from build123d import *

# Parameters (mm, degrees)
SKETCH4_R            = 8.5
SKETCH4_R_2          = 4.365
SKETCH4_R_3          = 3.8
SKETCH4_R_4          = 2.4
BOSS_EXTRUDE1_DEPTH  = 2
BOSS_EXTRUDE2_START  = 2
SKETCH4_3_R          = 8.5
SKETCH4_3_R_2        = 4.365
BOSS_EXTRUDE2_DEPTH  = 4
SKETCH4_4_R          = 2.4
CUT_EXTRUDE2_DEPTH   = 18.486852204
CUT_SWEEP1_PROFILE_R = 0.889
SKETCH14_R           = 2.75
SKETCH14_R_2         = 1.75
BOSS_EXTRUDE3_DEPTH  = 6
FILLET3_R            = 4
CHAMFER1_SIZE        = 1


with BuildPart() as part:
    # Sketch1 → Revolve1 (revolve)
    with BuildSketch(Plane(origin=(0, 0, 0), x_dir=(1, 0, 0), z_dir=(0, 1, 0))):
        Polygon((0, 0), (-12.7, 0), (-12.7, 4.365), (-8.73, 4.365), (-7.94, 5.155), (-7.15, 4.365), (-3.97, 4.365), (-3.97, 5.955), (0, 4.365), align=None)
    revolve(axis=Axis((0, 0, 0), (-1, 0, 0)))

    # Sketch4 → Boss-Extrude1 (add)
    # profile 1 of 3: a face of its own
    with BuildSketch(Plane.ZY.offset(12.7)):
        Circle(SKETCH4_R)
        with Locations(Location((0, 0, 0), (0, 0, 180))):
            Circle(SKETCH4_R_2, mode=Mode.SUBTRACT)
    # profile 2 of 3: a face of its own
    with BuildSketch(Plane.ZY.offset(12.7)):
        with Locations(Location((0, 0, 0), (0, 0, 180))):
            Circle(SKETCH4_R_2)
        Circle(SKETCH4_R_3, mode=Mode.SUBTRACT)
    # profile 3 of 3: a face of its own
    with BuildSketch(Plane.ZY.offset(12.7)):
        Circle(SKETCH4_R_3)
        Circle(SKETCH4_R_4, mode=Mode.SUBTRACT)
    extrude(amount=BOSS_EXTRUDE1_DEPTH)

    # Sketch4<3> → Boss-Extrude2 (add)
    with BuildSketch(Plane.ZY.offset(12.7).offset(BOSS_EXTRUDE2_START)):
        Circle(SKETCH4_3_R)
        with Locations(Location((0, 0, 0), (0, 0, 180))):
            Circle(SKETCH4_3_R_2, mode=Mode.SUBTRACT)
    extrude(amount=BOSS_EXTRUDE2_DEPTH)

    # Sketch4<4> → Cut-Extrude2 (cut, through all)
    with BuildSketch(Plane.ZY.offset(12.7)):
        Circle(SKETCH4_4_R)
    extrude(amount=-CUT_EXTRUDE2_DEPTH, mode=Mode.SUBTRACT)

    # Cut-Sweep1: sweep along a path in Sketch5
    with BuildLine(Plane.ZY.offset(18.7)) as cut_sweep1_path:
        CenterArc((0, 0), 6.082351302, 0, 360)
    # Cut-Sweep1 profile (on start of the path) → Cut-Sweep1 (sweep, cut)
    with BuildSketch(Plane(origin=(-18.7, 0, 6.082351302), x_dir=(0, 0, 1), z_dir=(0, 1, 0))):
        Circle(CUT_SWEEP1_PROFILE_R)
    sweep(path=cut_sweep1_path.line, mode=Mode.SUBTRACT)

    # Sketch14 → Boss-Extrude3 (add)
    # profile 1 of 3: a face of its own
    with BuildSketch(Plane.ZY.offset(18.7)):
        with Locations((10.5, 0)):
            Circle(SKETCH14_R)
        with Locations((10.5, 0)):
            Circle(SKETCH14_R_2, mode=Mode.SUBTRACT)
    # profile 2 of 3: a face of its own
    with BuildSketch(Plane.ZY.offset(18.7)):
        with Locations((-5.25, -9.09326674)):
            Circle(SKETCH14_R)
        with Locations((-5.25, -9.09326674)):
            Circle(SKETCH14_R_2, mode=Mode.SUBTRACT)
    # profile 3 of 3: a face of its own
    with BuildSketch(Plane.ZY.offset(18.7)):
        with Locations((-5.25, 9.09326674)):
            Circle(SKETCH14_R)
        with Locations((-5.25, 9.09326674)):
            Circle(SKETCH14_R_2, mode=Mode.SUBTRACT)
    extrude(amount=-BOSS_EXTRUDE3_DEPTH)

    # Fillet3
    # the kernel refuses this fillet: 4 mm, written as the material it adds along each edge
    with BuildSketch(Plane(origin=(-18.7, 8.059160345, -2.701839101), x_dir=(0, 0.13787930988752692, 0.9904490375102291), z_dir=(1, 0, 0))) as fillet3_piece_1:
        with BuildLine():
            CenterArc((3.866081399, -3.931630738), FILLET3_R, 100.608613334, 57.139697136)
            ThreePointArc((0.163964046, -2.4169271), (0.362452033, -1.189436498), (0, 0))
            ThreePointArc((0, 0), (1.564842471, -0.145284682), (3.129684942, 0))
        make_face()
    extrude(amount=6)
    with BuildSketch(Plane(origin=(-18.7, 6.369441471, -5.628518041), x_dir=(0, 0.559831667079214, -0.8286063628378122), z_dir=(1, 0, 0)), Plane(origin=(-18.7, -8.059160345, -2.701839101), x_dir=(0, -0.9975099934945784, -0.07052526411468515), z_dir=(1, 0, 0))) as fillet3_piece_2:
        with BuildLine():
            CenterArc((4.184287724, -3.591105941), FILLET3_R, 116.132681907, 57.139697136)
            ThreePointArc((0.211830564, -3.12250791), (0.250866796, -1.551420461), (0, 0))
            ThreePointArc((0, 0), (1.211241183, -0.281114665), (2.422482367, 0))
        make_face()
    extrude(amount=6)
    with BuildSketch(Plane(origin=(-18.7, -6.369441471, -5.628518041), x_dir=(0, -0.5598316670792142, -0.8286063628378122), z_dir=(1, 0, 0)), Plane(origin=(-18.7, -1.689718874, 8.330357143), x_dir=(0, -0.43767832641536075, 0.8991316269524996), z_dir=(1, 0, 0))) as fillet3_piece_3:
        with BuildLine():
            CenterArc((4.184287724, 3.591105941), FILLET3_R, 186.727620957, 57.139697136)
            ThreePointArc((0.211830564, 3.12250791), (0.250866796, 1.551420461), (0, 0))
            ThreePointArc((0, 0), (1.211241183, 0.281114665), (2.422482367, 0))
        make_face()
    extrude(amount=6)
    with BuildSketch(Plane(origin=(-18.7, 1.689718874, 8.330357143), x_dir=(0, 0.9266936825814681, -0.3758175337362501), z_dir=(1, 0, 0))) as fillet3_piece_4:
        with BuildLine():
            CenterArc((3.866081399, 3.931630738), FILLET3_R, 202.25168953, 57.139697136)
            ThreePointArc((0.163964046, 2.4169271), (0.362452033, 1.189436498), (0, 0))
            ThreePointArc((0, 0), (1.564842471, 0.145284682), (3.129684942, 0))
        make_face()
    extrude(amount=6)

    # Chamfer1
    chamfer1_edges = [part.edges().sort_by_distance(p)[0] for p in [
        (-14.7, 0, -2.4),
    ]]
    chamfer(chamfer1_edges, length=CHAMFER1_SIZE)


solid = part.part
Input: part model. Units: mm. Frame: model coordinates. A direction names the side the tool comes from. Round coordinates to 2 decimals unless told otherwise and drop trailing zeros. Order: outer loops, then holes, each group sorted by start corner. A loop starts at its lowest first (then second) coordinate and runs counter-clockwise, first axis right, second up. Notation, with made-up numbers: (-28, 68.25) - (0, 68.25) arc R10 ccw to (0, 86.25) - close; hole circle Ø8 at (-31.5, 74). An arc over 180 degrees is marked (long way). Answer as a JSON object with one key per item and string values. Group by question number.
(1) Cut plane C-C (y = 0). Count the separate pieces of the cut face and the enclosed holes in it, then the cut area to 3 significant figures.
(2) Material intervals for probe 1 along Y at (x, z) = (-16, -5.25); probe 2 along X at (y, z) = (-4.75, 0) (3 decimals); probe 3 along Z at (x, y) = (-14.75, 1), sorted ascending. Write a range as from..to.
(3) Reachability of faces 5 (the face through (-16.672, -4.328, 0.568)), 6 (the face through (-15.66, -7.39, 4.2)) from +Z, -Z, +X, -X, +Y, -Y: full face, straight path, thin tool, end or side. Return the list, or none.
(4) Draft query along X for faces 1 (the face through (-5.538, -2.95, 3.217)), 2 (the face through (-15.66, 7.33, 4.3)), 3 (the face through (-3.97, -4, 3)), 4 (the face through (0, 2, -2)). Return one class per face: released by +X, released by -X, zero draft, split by the parting line, or undercut.
(5) Pin query (flat end, axial travel): P1, Ø1.5, axis at x = -16, z = 3.5, coming from the +Y side; P2, Ø6, axis at x = -14, z = 0, coming from the -Y side; P3, Ø5, axis at y = 9, z = 3.5, coming from the +X side. Return the tip coordinate at first contact, or that it passes through.
(6) Cut plane A-A (z = 9.75). Return loops of the section in (x, y).
(7) Cut plane B-B (x = -4.75). Return loops of the section in (y, z) (3 decimals).
Here are the results:
{
 "1": {"separate pieces": "3", "enclosed holes": "0", "area": "119 mm^2"},
 "2": {"probe 1": "y = -11.84..-10.84, -7.34..7.34, 10.84..11.84", "probe 2": "x = -18.7..-12.7, -8.345..-7.535, -3.97..-0.961", "probe 3": "z = -8.44..-4.25, 4.25..9.06, 11.94..13.06"},
 "3": {"face 5": "-X", "face 6": "+Z, +X, -X, -Y"},
 "4": {"face 1": "undercut", "face 2": "zero draft", "face 3": "undercut", "face 4": "released by +X"},
 "5": {"P1": "stops at y = 8.04", "P2": "stops at y = -10.67", "P3": "stops at x = -12.7"},
 "6": {"outline": "(-18.7, -2.82) - (-12.7, -2.82) - (-12.7, -1.58) - (-18.7, -1.58) - close; (-18.7, 1.58) - (-12.7, 1.58) - (-12.7, 2.82) - (-18.7, 2.82) - close"},
 "7": {"outline": "circle Ø8.73 at (0, 0); hole circle Ø4.8 at (0, 0)"}
}
